Job drawing, mm, ordinate dimensions from the low corner. One solid piece. A direction names the side the tool comes from. Coordinates: 2 decimals unless noted, no trailing zeros. Loops run counter-clockwise (first coordinate to the right, second up) from the corner with the lowest first, then second, coordinate; pieces in that order, holes last. Notation, with made-up numbers: (10.25, 77) - (45.25, 77) arc R25 ccw to (45.25, 112) - close; hole circle Ø5 at (77.25, 11.5). An arc over 180 degrees is marked (long way). One line per question, with ' | ' between items. Start each with the question number.
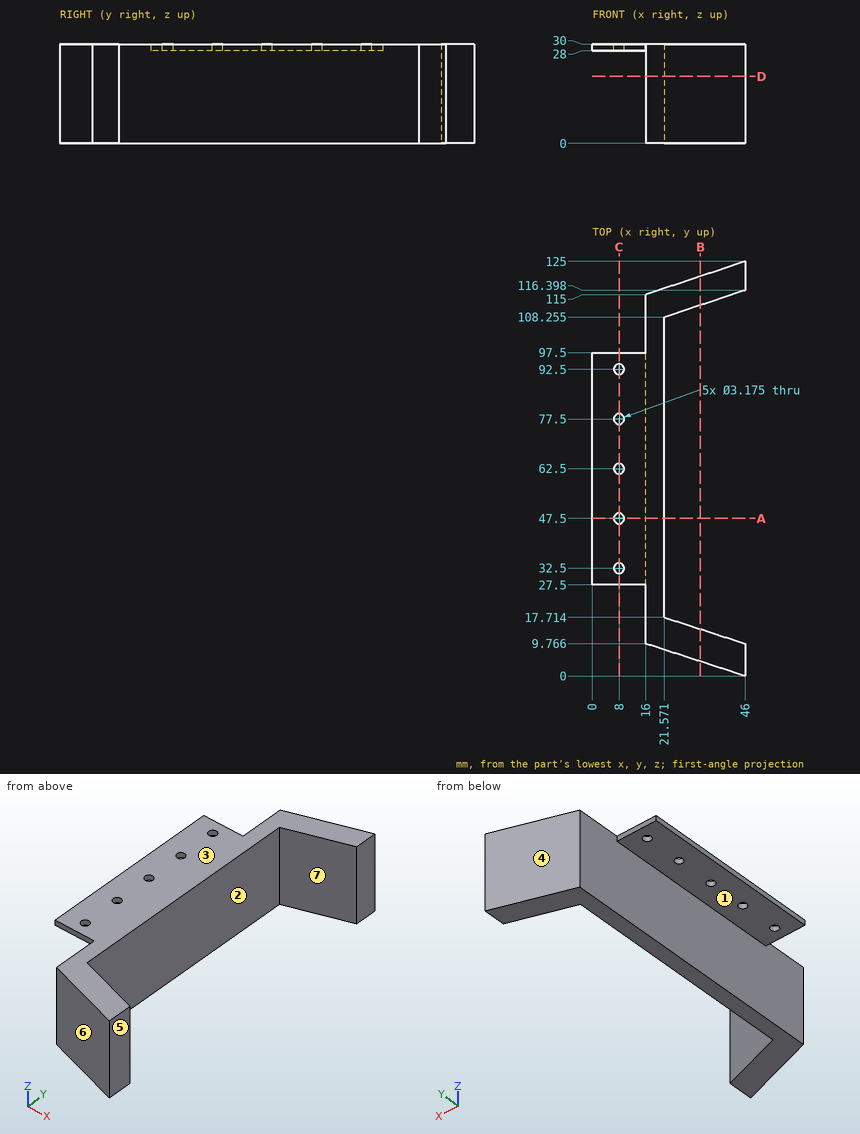
1) Band-saw the part on A-A on y = 47.5. List the corners of the cut face in (x, z), then the cut area to 3 significant figures.
2) Band-saw the part on D-D on z = 20.25. List the corners of the cut face in (x, y) (1 decimal).
3) Band-saw the part on C-C on x = 8. List the corners of the cut face in (y, z).
4) Mould opens along Y. For the marked faces 4, 5, 6 and 7 say: +Y half, -Y half, draft (parallel to the pull), parting line (faces both ways), or undercut.
5) Wall check: line 1 along X through (y, z) = (32.5, 28.6); line 2 along X through (y, z) = (30, 26.25); line 3 along Y through (x, z) = (23.5, 8) (1 decimal). Give the ranges that are in metal, low to high. Write a range as [from, to].
6) Band-saw the part on B-B on x = 32.5. List the corners of the cut face in (y, z) (1 decimal), then the cut area to 3 significant figures.
7) Tool access for the marked faces 1, 2 and 3: list every direction of +Z, -Z, +X, -X, +Y, -Y with a clear straight run to the whole face (end or side of a thin tool).
8) Pin check, flat tips, straight feed: pin 1 Ø4 at (x, y) = (8, 92.5) entering from -Z; pin 2 Ø4 at (x, z) = (19.5, 18) entering from +Y; pin 3 Ø10 at (y, z) = (33, 22) entering from +X. Stop position of each tip, or through.
Values found:
1) outline: (0, 28) - (6.41, 28) - (6.41, 30) - (0, 30) - close; (9.59, 28) - (16, 28) - (16, 0) - (21.57, 0) - (21.57, 30) - (9.59, 30) - close | area: 193 mm²
2) outline: (16, 9.8) - (46, 0) - (46, 9.8) - (21.6, 17.7) - (21.6, 108.3) - (46, 116.4) - (46, 125) - (16, 115) - close
3) outline: (27.5, 28) - (30.91, 28) - (30.91, 30) - (27.5, 30) - close; (34.09, 28) - (45.91, 28) - (45.91, 30) - (34.09, 30) - close; (49.09, 28) - (60.91, 28) - (60.91, 30) - (49.09, 30) - close; (64.09, 28) - (75.91, 28) - (75.91, 30) - (64.09, 30) - close; (79.09, 28) - (90.91, 28) - (90.91, 30) - (79.09, 30) - close; (94.09, 28) - (97.5, 28) - (97.5, 30) - (94.09, 30) - close
4) face 4: +Y half | face 5: draft | face 6: -Y half | face 7: undercut
5) line 1: [0, 6.41], [9.59, 21.57] | line 2: [16, 21.57] | line 3: [7.3, 17.1], [108.9, 117.5]
6) outline: (4.4, 0) - (14.2, 0) - (14.2, 30) - (4.4, 30) - close; (111.9, 0) - (120.5, 0) - (120.5, 30) - (111.9, 30) - close | area: 551 mm²
7) face 1: -Z, -X, +Y, -Y | face 2: +Z, -Z, +X | face 3: +Z, +X, -X, +Y, -Y
8) pin 1: z = 28 | pin 2: y = 116.83 | pin 3: x = 21.57
